```python
from build123d import *

# Parameters (mm, degrees)
EXTRUDE_THIN1_START          = -19.05
EXTRUDE_THIN1_DEPTH          = 38.1
SKETCH4_R                    = 2.0828
EXTRUDE3_DEPTH               = 74.291654886
SKETCH5_R                    = 2.0828
CUT_EXTRUDE1_DEPTH           = 2.54
CUT_EXTRUDE1_DRAFT           = 41
CUT_EXTRUDE1_PROFILE_2_DEPTH = 2.54
CUT_EXTRUDE1_PROFILE_2_DRAFT = 41
CUT_EXTRUDE1_PROFILE_3_DEPTH = 2.54
CUT_EXTRUDE1_PROFILE_3_DRAFT = 41
MIRROR1_COPY_1_SKETCH_R      = 2.0828
MIRROR1_COPY_1_DEPTH         = 2.54
MIRROR1_COPY_1_DRAFT         = 41
MIRROR1_COPY_2_SKETCH_R      = 2.0828
MIRROR1_COPY_2_DEPTH         = 2.54
MIRROR1_COPY_2_DRAFT         = 41
MIRROR1_COPY_3_SKETCH_R      = 2.0828
MIRROR1_COPY_3_DEPTH         = 2.54
MIRROR1_COPY_3_DRAFT         = 41
MIRROR1_COPY_4_SKETCH_R      = 2.0828
MIRROR1_COPY_4_DEPTH         = 2.54
MIRROR1_COPY_4_DRAFT         = 41
MIRROR1_COPY_5_SKETCH_R      = 2.0828
MIRROR1_COPY_5_DEPTH         = 2.54
MIRROR1_COPY_5_DRAFT         = 41


# Read off the part's stored shape, not the designer's step: Extrude-Thin1
with BuildPart() as part:
    # Extrude-Thin1 outline → Extrude-Thin1 (new body)
    with BuildSketch(Plane(origin=(0, 0, 0), x_dir=(1, 0, 0), z_dir=(0, 1, 0)).offset(EXTRUDE_THIN1_START)):
        with BuildLine():
            Line((2.286, -1.524), (50.8, -1.524))
            Line((50.8, -1.524), (50.8, 0))
            Line((50.8, 0), (2.286, 0))
            ThreePointArc((2.286, 0), (0.669553898, -0.669553898), (0, -2.286))
            Line((0, -2.286), (0, -50.8))
            Line((0, -50.8), (1.524, -50.8))
            Line((1.524, -50.8), (1.524, -2.286))
            ThreePointArc((1.524, -2.286), (1.747184633, -1.747184633), (2.286, -1.524))
        make_face()
    extrude(amount=EXTRUDE_THIN1_DEPTH)

    # Sketch4 → Extrude3 (cut, through all)
    with BuildSketch(Plane(origin=(1.524, 0, 0), x_dir=(0, 0, -1), z_dir=(1, 0, 0))):
        with Locations((-41.275, 0)):
            Circle(SKETCH4_R)
        with Locations((-22.225, 12.7)):
            Circle(SKETCH4_R)
        with Locations((-22.225, -12.7)):
            Circle(SKETCH4_R)
    extrude3 = extrude(amount=-EXTRUDE3_DEPTH, mode=Mode.SUBTRACT)


with BuildPart() as cut_extrude1_tool:
    # Sketch5 → Cut-Extrude1 (with draft: the straight prism first)
    with BuildSketch(Plane.ZY):
        with Locations((22.225, -12.7)):
            Circle(SKETCH5_R)
    extrude(amount=-CUT_EXTRUDE1_DEPTH)
    # Cut-Extrude1: the draft: its side faces are tilted about the plane it starts from
    cut_extrude1_sides = [cut_extrude1_tool.faces().sort_by_distance(p)[0] for p in [
        (1.27, -12.7, 20.1422),
    ]]
    draft(cut_extrude1_sides, Plane.ZY, CUT_EXTRUDE1_DRAFT)


with BuildPart() as part_1:
    add(part.part)

    # Cut-Extrude1: cut by cut_extrude1_tool
    add(cut_extrude1_tool.part, mode=Mode.SUBTRACT)


with BuildPart() as cut_extrude1_profile_2_tool:
    # Sketch5 → Cut-Extrude1 profile 2 (with draft: the straight prism first)
    with BuildSketch(Plane.ZY):
        with Locations((22.225, 12.7)):
            Circle(SKETCH5_R)
    extrude(amount=-CUT_EXTRUDE1_PROFILE_2_DEPTH)
    # Cut-Extrude1 profile 2: the draft: its side faces are tilted about the plane it starts from
    cut_extrude1_profile_2_sides = [cut_extrude1_profile_2_tool.faces().sort_by_distance(p)[0] for p in [
        (1.27, 12.7, 20.1422),
    ]]
    draft(cut_extrude1_profile_2_sides, Plane.ZY, CUT_EXTRUDE1_PROFILE_2_DRAFT)


with BuildPart() as part_2:
    add(part_1.part)

    # Cut-Extrude1 profile 2: cut by cut_extrude1_profile_2_tool
    add(cut_extrude1_profile_2_tool.part, mode=Mode.SUBTRACT)


with BuildPart() as cut_extrude1_profile_3_tool:
    # Sketch5 → Cut-Extrude1 profile 3 (with draft: the straight prism first)
    with BuildSketch(Plane.ZY):
        with Locations((41.275, 0)):
            Circle(SKETCH5_R)
    extrude(amount=-CUT_EXTRUDE1_PROFILE_3_DEPTH)
    # Cut-Extrude1 profile 3: the draft: its side faces are tilted about the plane it starts from
    cut_extrude1_profile_3_sides = [cut_extrude1_profile_3_tool.faces().sort_by_distance(p)[0] for p in [
        (1.27, 0, 39.1922),
    ]]
    draft(cut_extrude1_profile_3_sides, Plane.ZY, CUT_EXTRUDE1_PROFILE_3_DRAFT)


with BuildPart() as part_3:
    add(part_2.part)

    # Cut-Extrude1 profile 3: cut by cut_extrude1_profile_3_tool
    add(cut_extrude1_profile_3_tool.part, mode=Mode.SUBTRACT)

    # Mirror1: Extrude3 across plane
    add(extrude3.mirror(Plane(origin=(0, 0, 0), x_dir=(0.7071067811865465, 0, 0.7071067811865486), z_dir=(-0.7071067811865488, 0, 0.7071067811865464))), mode=Mode.SUBTRACT)


with BuildPart() as mirror1_copy_1_tool:
    # Mirror1 copy 1 sketch → Mirror1 copy 1 (with draft: the straight prism first)
    with BuildSketch(Plane(origin=(0, 0, 0), x_dir=(1, 0, 0), z_dir=(0, 0, -1))):
        with Locations((22.225, 12.7)):
            Circle(MIRROR1_COPY_1_SKETCH_R)
    extrude(amount=-MIRROR1_COPY_1_DEPTH)
    # Mirror1 copy 1: the draft: its side faces are tilted about the plane it starts from
    mirror1_copy_1_sides = [mirror1_copy_1_tool.faces().sort_by_distance(p)[0] for p in [
        (20.1422, -12.7, 1.27),
    ]]
    draft(mirror1_copy_1_sides, Plane(origin=(0, 0, 0), x_dir=(1, 0, 0), z_dir=(0, 0, -1)), MIRROR1_COPY_1_DRAFT)


with BuildPart() as part_4:
    add(part_3.part)

    # Mirror1 copy 1: cut by mirror1_copy_1_tool
    add(mirror1_copy_1_tool.part, mode=Mode.SUBTRACT)


with BuildPart() as mirror1_copy_2_tool:
    # Mirror1 copy 2 sketch → Mirror1 copy 2 (with draft: the straight prism first)
    with BuildSketch(Plane(origin=(0, 0, 0), x_dir=(1, 0, 0), z_dir=(0, 0, -1))):
        with Locations((22.225, -12.7)):
            Circle(MIRROR1_COPY_2_SKETCH_R)
    extrude(amount=-MIRROR1_COPY_2_DEPTH)
    # Mirror1 copy 2: the draft: its side faces are tilted about the plane it starts from
    mirror1_copy_2_sides = [mirror1_copy_2_tool.faces().sort_by_distance(p)[0] for p in [
        (20.1422, 12.7, 1.27),
    ]]
    draft(mirror1_copy_2_sides, Plane(origin=(0, 0, 0), x_dir=(1, 0, 0), z_dir=(0, 0, -1)), MIRROR1_COPY_2_DRAFT)


with BuildPart() as part_5:
    add(part_4.part)

    # Mirror1 copy 2: cut by mirror1_copy_2_tool
    add(mirror1_copy_2_tool.part, mode=Mode.SUBTRACT)


with BuildPart() as mirror1_copy_3_tool:
    # Mirror1 copy 3 sketch → Mirror1 copy 3 (with draft: the straight prism first)
    with BuildSketch(Plane(origin=(0, 0, 0), x_dir=(1, 0, 0), z_dir=(0, 0, -1))):
        with Locations((41.275, 0)):
            Circle(MIRROR1_COPY_3_SKETCH_R)
    extrude(amount=-MIRROR1_COPY_3_DEPTH)
    # Mirror1 copy 3: the draft: its side faces are tilted about the plane it starts from
    mirror1_copy_3_sides = [mirror1_copy_3_tool.faces().sort_by_distance(p)[0] for p in [
        (39.1922, 0, 1.27),
    ]]
    draft(mirror1_copy_3_sides, Plane(origin=(0, 0, 0), x_dir=(1, 0, 0), z_dir=(0, 0, -1)), MIRROR1_COPY_3_DRAFT)


with BuildPart() as part_6:
    add(part_5.part)

    # Mirror1 copy 3: cut by mirror1_copy_3_tool
    add(mirror1_copy_3_tool.part, mode=Mode.SUBTRACT)


with BuildPart() as mirror1_copy_4_tool:
    # Mirror1 copy 4 sketch → Mirror1 copy 4 (with draft: the straight prism first)
    with BuildSketch(Plane(origin=(0, 0, 0), x_dir=(1, 0, 0), z_dir=(0, 0, -1))):
        with Locations((22.225, -12.7)):
            Circle(MIRROR1_COPY_4_SKETCH_R)
    extrude(amount=-MIRROR1_COPY_4_DEPTH)
    # Mirror1 copy 4: the draft: its side faces are tilted about the plane it starts from
    mirror1_copy_4_sides = [mirror1_copy_4_tool.faces().sort_by_distance(p)[0] for p in [
        (20.1422, 12.7, 1.27),
    ]]
    draft(mirror1_copy_4_sides, Plane(origin=(0, 0, 0), x_dir=(1, 0, 0), z_dir=(0, 0, -1)), MIRROR1_COPY_4_DRAFT)


with BuildPart() as part_7:
    add(part_6.part)

    # Mirror1 copy 4: cut by mirror1_copy_4_tool
    add(mirror1_copy_4_tool.part, mode=Mode.SUBTRACT)


with BuildPart() as mirror1_copy_5_tool:
    # Mirror1 copy 5 sketch → Mirror1 copy 5 (with draft: the straight prism first)
    with BuildSketch(Plane(origin=(0, 0, 0), x_dir=(1, 0, 0), z_dir=(0, 0, -1))):
        with Locations((41.275, 0)):
            Circle(MIRROR1_COPY_5_SKETCH_R)
    extrude(amount=-MIRROR1_COPY_5_DEPTH)
    # Mirror1 copy 5: the draft: its side faces are tilted about the plane it starts from
    mirror1_copy_5_sides = [mirror1_copy_5_tool.faces().sort_by_distance(p)[0] for p in [
        (39.1922, 0, 1.27),
    ]]
    draft(mirror1_copy_5_sides, Plane(origin=(0, 0, 0), x_dir=(1, 0, 0), z_dir=(0, 0, -1)), MIRROR1_COPY_5_DRAFT)


with BuildPart() as part_8:
    add(part_7.part)

    # Mirror1 copy 5: cut by mirror1_copy_5_tool
    add(mirror1_copy_5_tool.part, mode=Mode.SUBTRACT)


solid = part_8.part
```
The listing builds one solid part. Answer for the finished solid, in the listing's coordinates (mm). A direction names the side the tool comes from. Coordinates: 2 decimals unless noted, no trailing zeros. Write each loop counter-clockwise with the first axis right and the second up, starting at its lowest first coordinate (ties: lowest second). Pieces come first, ordered by that corner, then holes. Notation, with made-up numbers: (82, 5) - (102, 5) arc R26 ccw to (102, 21) - close; hole circle Ø3 at (67, 52). An arc over 180 degrees is marked (long way). Return JSON: item names as keys, results as strings. Group by question number.
1. A cutting plane is placed at C-C, the plane y = 0. Determine the outline of the cut face in (x, z), plus the area to 3 significant figures.
2. A cutting plane is placed at D-D, the plane z = 4. Determine the outline of the cut face in (x, y), plus the area to 3 significant figures.
3. Which of the six approach directions +Z, -Z, +X, -X, +Y, -Y give full straight-line access (tool end or side, diameter ignored) to faces 1 (the flat face through (26, 0, 1.524)), 2 (the flat face through (50.8, 0, 1))?
4. Given pin 1 (8 mm diameter, centred on x = 24, y = -9.5, fed in from +Z); pin 2 (10 mm diameter, centred on y = -0.5, z = 9.5, fed in from +X); pin 3 (12 mm diameter, centred on y = -8, z = 20, fed in from -X), each flat-ended and moving along its own axis, determine where each tip first touches the part or whether it passes through.
5. A cutting plane is placed at B-B, the plane x = 35.5. Determine the outline of the cut face in (y, z).
6. A cutting plane is placed at A-A, the plane y = 7.5. Determine the outline of the cut face in (x, z).
7. Straight lines are drawn through the part: L1, parallel to Z at x = 34, y = -12.5; L2, parallel to Z at x = 20, y = -10.5. For each, find the intervals that lie inside material, in ascending order.
Ans:
{
 "1": {"outline": "(0, 2.29) arc R2.29 ccw to (2.29, 0) - (39.19, 0) - (37.87, 1.52) - (2.29, 1.52) arc R0.76 cw to (1.52, 2.29) - (1.52, 37.87) - (0, 39.19) - close; (0, 43.36) - (1.52, 44.68) - (1.52, 50.8) - (0, 50.8) - close; (43.36, 0) - (50.8, 0) - (50.8, 1.52) - (44.68, 1.52) - close", "area": "135 mm²"},
 "2": {"outline": "(0, -19.05) - (1.52, -19.05) - (1.52, 19.05) - (0, 19.05) - close", "area": "58.1 mm²"},
 "3": {"face 1": "+Z, +X, +Y, -Y", "face 2": "+Z, -Z, +X, +Y, -Y"},
 "4": {"pin 1": "z = 1.52", "pin 2": "x = 1.52", "pin 3": "x = 0"},
 "5": {"outline": "(-19.05, 0) - (19.05, 0) - (19.05, 1.52) - (-19.05, 1.52) - close"},
 "6": {"outline": "(0, 2.29) arc R2.29 ccw to (2.29, 0) - (50.8, 0) - (50.8, 1.52) - (2.29, 1.52) arc R0.76 cw to (1.52, 2.29) - (1.52, 50.8) - (0, 50.8) - close"},
 "7": {"L1": "0 to 1.52", "L2": "0 to 1.2"}
}
